```python
from build123d import *

# Parameters (mm, degrees)
SKETCH1_R           = 10
BOSS_EXTRUDE1_DEPTH = 10


with BuildPart() as part:
    # Sketch1 → Boss-Extrude1 (new, symmetric)
    with BuildSketch(Plane.XY):
        with BuildLine():
            Line((23.804506832, 7.638419634), (12, 50))
            ThreePointArc((12, 50), (0, 62), (-12, 50))
            Line((-12, 50), (-23.804506832, 7.638419634))
            Line((-23.804506832, 7.638419634), (-24.324275855, 5.773179723))
            ThreePointArc((-24.324275855, 5.773179723), (-24.754655731, 3.49385455), (-24.971925744, 1.184451201))
            ThreePointArc((-24.971925744, 1.184451201), (-32.933355329, -17.072864969), (-51.021497025, -25.411515024))
            ThreePointArc((-51.021497025, -25.411515024), (-60.239080638, -51.338500415), (-35, -40.376692732))
            ThreePointArc((-35, -40.376692732), (-26.790738996, -24.957326865), (-9.41500118, -23.1593988))
            ThreePointArc((-9.41500118, -23.1593988), (0, -25), (9.41500118, -23.1593988))
            ThreePointArc((9.41500118, -23.1593988), (26.790738996, -24.957326865), (35, -40.376692732))
            ThreePointArc((35, -40.376692732), (60.239080638, -51.338500415), (51.021497025, -25.411515024))
            ThreePointArc((51.021497025, -25.411515024), (32.933355329, -17.072864969), (24.971925744, 1.184451201))
            ThreePointArc((24.971925744, 1.184451201), (24.754655731, 3.49385455), (24.324275855, 5.773179723))
            Line((24.324275855, 5.773179723), (23.804506832, 7.638419634))
        make_face()
        with Locations((-50, -40.376692732)):
            Circle(SKETCH1_R, mode=Mode.SUBTRACT)
        with Locations((50, -40.376692732)):
            Circle(SKETCH1_R, mode=Mode.SUBTRACT)
        with BuildLine():
            ThreePointArc((-5, 50), (0, 55), (5, 50))
            Line((5, 50), (19.048602886, 6.095139711))
            ThreePointArc((19.048602886, 6.095139711), (0, -20), (-19.048602886, 6.095139711))
            Line((-19.048602886, 6.095139711), (-5, 50))
        make_face(mode=Mode.SUBTRACT)
    extrude(amount=BOSS_EXTRUDE1_DEPTH, both=True)


solid = part.part
```
Source: CAD feature listing. Evaluate the final solid. Frame: model axes, mm. A direction names the side the tool comes from. Round coordinates to 2 decimals unless told otherwise and drop trailing zeros. Loops run counter-clockwise (first coordinate to the right, second up) from the corner with the lowest first, then second, coordinate; pieces in that order, holes last.
(1) Section query C-C (z = 4). Output: boundary loops of the cut face in (x, y) (1 decimal).
From the geometry:
outline: (-51, -25.4) arc R15 ccw (long way) to (-35, -40.4) arc R18.6 cw to (-9.4, -23.2) arc R25 ccw to (9.4, -23.2) arc R18.6 cw to (35, -40.4) arc R15 ccw (long way) to (51, -25.4) arc R28 cw to (25, 1.2) arc R25 ccw to (24.3, 5.8) - (12, 50) arc R12 ccw to (-12, 50) - (-24.3, 5.8) arc R25 ccw to (-25, 1.2) arc R28 cw to start; hole circle Ø20 at (-50, -40.4); hole (-19, 6.1) arc R20 ccw (long way) to (19, 6.1) - (5, 50) arc R5 ccw to (-5, 50) - close; hole circle Ø20 at (50, -40.4)
(2) Contact query for flat-ended pins moving along their axis: pin 1 Ø1.5 at (x, z) = (-20.5, -5) entering from -Y; pin 2 Ø1 at (x, z) = (-36.5, 6.5) entering from -Y; pin 3 Ø1 at (x, z) = (28, -2.5) entering from -Y. Output: stop coordinate, or through.
From the geometry:
pin 1: stops at y = -22.43
pin 2: stops at y = -47.86
pin 3: stops at y = -26.26
(3) Pull-direction query (Y, two-part tool) for faces 1 (the flat face through (-10, -18, -10)), 2 (the cylindrical face through (-59.99, -39.94, -0.14)), 3 (the cylindrical face through (24.76, 3.46, 0.14)); classes: +Y half, -Y half, draft (parallel to the pull), parting line (faces both ways), or undercut.
From the geometry:
face 1: draft
face 2: undercut
face 3: +Y half
(4) Section query B-B (y = 25.5). Output: boundary loops of the cut face in (x, z), and give its area (3 significant figures).
From the geometry:
outline: (-18.83, -10) - (-12.84, -10) - (-12.84, 10) - (-18.83, 10) - close; (12.84, -10) - (18.83, -10) - (18.83, 10) - (12.84, 10) - close
area: 240 mm2
(5) Access query for faces 4 (the cylindrical face through (0, 62, 0)), 5 (the flat face through (11.926, 28.355, 0.14)). Directions: +Z, -Z, +X, -X, +Y, -Y. A direction counts if a zero-diameter tool reaches every point of the face in a straight line with its end or side. Return the directions, or none.
From the geometry:
face 4: +Z, -Z, +Y
face 5: +Z, -Z
(6) Section query A-A (x = 0). Output: boundary loops of the cut face in (y, z).
From the geometry:
outline: (-25, -10) - (-20, -10) - (-20, 10) - (-25, 10) - close; (55, -10) - (62, -10) - (62, 10) - (55, 10) - close
(7) Material intervals for probe 1 along X at (y, z) = (-40, 6.5); probe 2 along X at (y, z) = (0, 3.5); probe 3 along X at (y, z) = (36, -5), sorted ascending.
From the geometry:
probe 1: x = -65 to -59.99, -40.01 to -35, 35 to 40.01, 59.99 to 65
probe 2: x = -25.05 to -20, 20 to 25.05
probe 3: x = -15.9 to -9.48, 9.48 to 15.9
